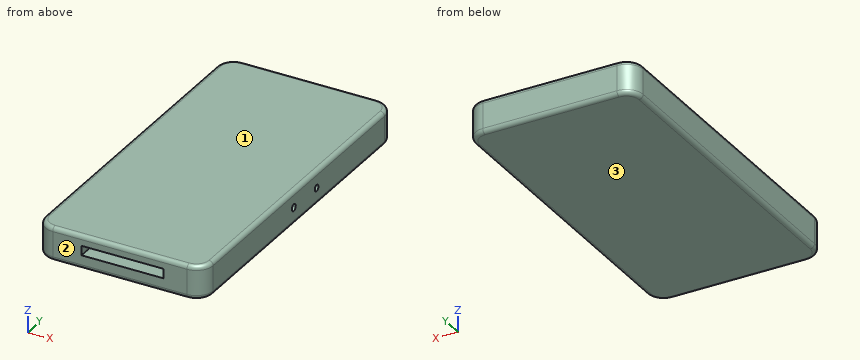
```python
from build123d import *

# Parameters (mm, degrees)
F0_W     = 40
F0_H     = 80
F1_DEPTH = 8
F2_R     = 4
F3_R     = 1
F4_W     = 19.56314
F4_H     = 2.266603
F5_DEPTH = 5
F6_R     = 0.760622
F6_R_2   = 0.822373
F7_DEPTH = 5


with BuildPart() as f1:
    # F0 (on Top) → F1 (new body)
    with BuildSketch(Plane.XY):
        with Locations((-15.960967, 3.776696)):
            Rectangle(F0_W, F0_H)
    extrude(amount=F1_DEPTH)

    # F2
    f2_edges = [f1.edges().sort_by_distance(p)[0] for p in [
        (4.039033, 43.776696, 4),
        (4.039033, -36.223304, 4),
        (-35.960967, -36.223304, 4),
        (-35.960967, 43.776696, 4),
    ]]
    fillet(f2_edges, radius=F2_R)

    # F3
    f3_edges = [f1.edges().sort_by_distance(p)[0] for p in [
        (-35.960967, 3.776696, 8),
        (-35.960967, 3.776696, 0),
    ]]
    fillet(f3_edges, radius=F3_R)

    # F4 (on face) → F5 (cut)
    with BuildSketch(Plane.XZ.offset(36.223304)):
        with Locations((-15.319868, 4.395118)):
            Rectangle(F4_W, F4_H)
    extrude(amount=-F5_DEPTH, mode=Mode.SUBTRACT)

    # F6 (on face) → F7 (cut)
    with BuildSketch(Plane.YZ.offset(4.039033)):
        with Locations((11.231415, 3.99991)):
            Circle(F6_R)
        with Locations((1.659386, 4.084856)):
            Circle(F6_R_2)
    extrude(amount=-F7_DEPTH, mode=Mode.SUBTRACT)


solid = f1.part
```
Input: part model. Units: mm. Frame: model coordinates. Face numbers are marked on the shaded views. Coordinates: 2 decimals unless noted, no trailing zeros. Loops run counter-clockwise (first coordinate to the right, second up) from the corner with the lowest first, then second, coordinate; pieces in that order, holes last. Notation, with made-up numbers: M 30,-25 L 58,-25 A8 ccw 58,-21 Z; hole C 32.25,60.5 d7. An arc over 180 degrees is marked long. Use a Markdown table: item, result. Add a question column.
1) Line query: L1, parallel to Y at x = -10, z = 3.5; L2, parallel to Y at x = -4.5, z = 7.5; L3, parallel to X at y = -28, z = 0.75. Output: solid intervals per line, ascending. Write a range as from..to.
2) Section A-A, the plane x = -8. Return the cut outline in (y, z), plus the area to 3 significant figures.
3) Pin query (flat end, axial travel): P1, Ø0.7, axis at y = -34, z = 4.5, coming from the +X side; P2, Ø0.7, axis at x = -20, z = 4, coming from the -Y side; P3, Ø1.1, axis at y = -35, z = 4.5, coming from the -X side. Return the tip coordinate at first contact, or that it passes through.
4) Draft query along Z for the marked faces 1, 2 and 3. Return one class per face: +Z half, -Z half, draft (parallel to the pull), parting line (faces both ways), or undercut.
Answer below:
| question | item | result |
|---|---|---|
| 1 | L1 | -31.22..43.78 |
| 1 | L2 | -36.09..43.64 |
| 1 | L3 | -35.93..4.01 |
| 2 | outline | M -36.22,1 A1 ccw -35.22,0 L 42.78,0 A1 ccw 43.78,1 L 43.78,7 A1 ccw 42.78,8 L -35.22,8 A1 ccw -36.22,7 L -36.22,5.53 L -31.22,5.53 L -31.22,3.26 L -36.22,3.26 Z |
| 2 | area | 628 mm2 |
| 3 | P1 | x = 3.78 |
| 3 | P2 | y = -31.22 |
| 3 | P3 | x = -35.28 |
| 4 | face 1 | +Z half |
| 4 | face 2 | draft |
| 4 | face 3 | -Z half |
